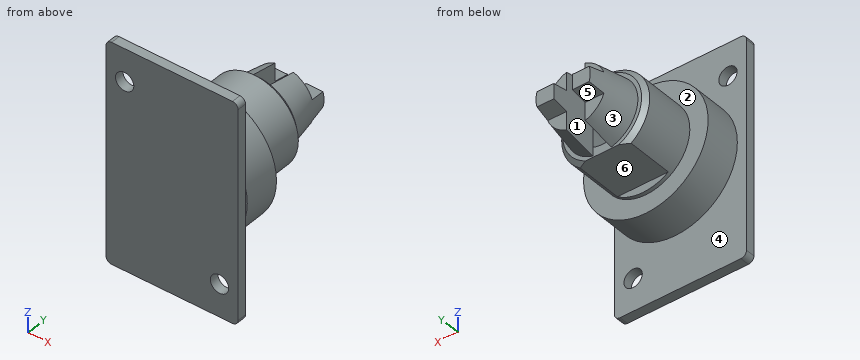
from build123d import *

# Parameters (mm, degrees)
BOSS_EXTRUDE1_DEPTH     = 1.27
SKETCH3_W               = 12
SKETCH3_H               = 12
CUT_EXTRUDE1_DEPTH      = 6.985
CUT_EXTRUDE1_DEPTH_BACK = 6.985
CUT_EXTRUDE2_DEPTH      = 12
CUT_EXTRUDE2_DEPTH_BACK = 12
SKETCH6_W               = 9.7536
SKETCH6_H               = 7.3914
CUT_EXTRUDE3_DEPTH      = 1.27
CUT_EXTRUDE3_DEPTH_BACK = 1.27
SKETCH7_R               = 1.25
CUT_EXTRUDE4_DEPTH      = 2.54
CUT_EXTRUDE4_DEPTH_BACK = 2.54
SKETCH8_R               = 1.25
CUT_EXTRUDE5_DEPTH      = 2.54
CUT_EXTRUDE5_DEPTH_BACK = 2.54


with BuildPart() as part:
    # Sketch1 → Boss-Extrude1 (new body)
    with BuildSketch(Plane(origin=(0, 0, 0), x_dir=(1, 0, 0), z_dir=(0, 1, 0))):
        with BuildLine():
            Line((-9.0043, 14.2367), (-9.0043, -14.2367))
            ThreePointArc((-9.0043, -14.2367), (-8.781115367, -14.775515367), (-8.2423, -14.9987))
            Line((-8.2423, -14.9987), (8.2423, -14.9987))
            ThreePointArc((8.2423, -14.9987), (8.781115367, -14.775515367), (9.0043, -14.2367))
            Line((9.0043, -14.2367), (9.0043, 14.2367))
            ThreePointArc((9.0043, 14.2367), (8.781115367, 14.775515367), (8.2423, 14.9987))
            Line((8.2423, 14.9987), (-8.2423, 14.9987))
            ThreePointArc((-8.2423, 14.9987), (-8.781115367, 14.775515367), (-9.0043, 14.2367))
        make_face()
    extrude(amount=BOSS_EXTRUDE1_DEPTH)

    # Sketch2 → Revolve1 (revolve)
    with BuildSketch(Plane(origin=(0, 0, 0), x_dir=(0, 0, -1), z_dir=(1, 0, 0))):
        Polygon((3.7592, 14.7066), (3.7592, 0.9398), (6.589242136, 0.9398), (6.126999938, 2.2098), (8.4963, 2.2098), (8.4963, 7.2136), (5.999999938, 7.2136), (5.999999938, 14.093100062), (5.3865, 14.7066), align=None)
    revolve(axis=Axis((0, 0.9398, 0), (0, 1, 0)))

    # Sketch3 → Cut-Extrude1 (cut, two sides)
    with BuildSketch(Plane(origin=(0, 14.7066, 0), x_dir=(1, 0, 0), z_dir=(0, 1, 0))) as cut_extrude1_sk:
        with Locations((0, 10.8966)):
            Rectangle(SKETCH3_W, SKETCH3_H)
    extrude(amount=CUT_EXTRUDE1_DEPTH, mode=Mode.SUBTRACT)
    extrude(cut_extrude1_sk.sketch, amount=-CUT_EXTRUDE1_DEPTH_BACK, mode=Mode.SUBTRACT)

    # Sketch4 → Revolve2 (revolve)
    with BuildSketch(Plane(origin=(0, 0, 0), x_dir=(0, 0, -1), z_dir=(1, 0, 0))):
        Polygon((0, 22.098), (3.573496755, 22.098), (4.8768, 14.7066), (0, 14.7066), align=None)
    revolve(axis=Axis((0, 14.7066, 0), (0, 1, 0)))

    # Sketch5 → Cut-Extrude2 (cut, two sides)
    with BuildSketch(Plane(origin=(0, 0, 0), x_dir=(0, 0, -1), z_dir=(1, 0, 0))) as cut_extrude2_sk:
        Polygon((-4.8768, 23.6982), (-4.08406916, 19.2024), (-1.418134328, 19.2024), (-1.032965672, 21.3868), (1.032965672, 21.3868), (1.418134328, 19.2024), (4.08406916, 19.2024), (4.8768, 23.6982), align=None)
    extrude(amount=CUT_EXTRUDE2_DEPTH, mode=Mode.SUBTRACT)
    extrude(cut_extrude2_sk.sketch, amount=-CUT_EXTRUDE2_DEPTH_BACK, mode=Mode.SUBTRACT)

    # Sketch6 → Cut-Extrude3 (cut, two sides)
    with BuildSketch(Plane(origin=(0, 0, 0), x_dir=(0, 0, -1), z_dir=(1, 0, 0))) as cut_extrude3_sk:
        with Locations((0, 18.4023)):
            Rectangle(SKETCH6_W, SKETCH6_H)
    extrude(amount=CUT_EXTRUDE3_DEPTH, mode=Mode.SUBTRACT)
    extrude(cut_extrude3_sk.sketch, amount=-CUT_EXTRUDE3_DEPTH_BACK, mode=Mode.SUBTRACT)

    # Sketch7 → Cut-Extrude4 (cut, two sides)
    with BuildSketch(Plane(origin=(0, 0, 0), x_dir=(1, 0, 0), z_dir=(0, 1, 0))) as cut_extrude4_sk:
        with Locations((6.4643, 10.541)):
            Circle(SKETCH7_R)
    extrude(amount=CUT_EXTRUDE4_DEPTH, mode=Mode.SUBTRACT)
    extrude(cut_extrude4_sk.sketch, amount=-CUT_EXTRUDE4_DEPTH_BACK, mode=Mode.SUBTRACT)

    # Sketch8 → Cut-Extrude5 (cut, two sides)
    with BuildSketch(Plane(origin=(0, 0, 0), x_dir=(1, 0, 0), z_dir=(0, 1, 0))) as cut_extrude5_sk:
        with Locations((-6.4643, -10.541)):
            Circle(SKETCH8_R)
    extrude(amount=CUT_EXTRUDE5_DEPTH, mode=Mode.SUBTRACT)
    extrude(cut_extrude5_sk.sketch, amount=-CUT_EXTRUDE5_DEPTH_BACK, mode=Mode.SUBTRACT)


solid = part.part
Input: part model. Units: mm. Frame: model coordinates. Face numbers are marked on the shaded views. A direction names the side the tool comes from. Coordinates: 2 decimals unless noted, no trailing zeros. Loops run counter-clockwise (first coordinate to the right, second up) from the corner with the lowest first, then second, coordinate; pieces in that order, holes last. Notation, with made-up numbers: (-23.5, 80) -> (17.5, 80) arc R19 cw to (17.5, 98) -> close; hole circle Ø11 at (27.25, -37). An arc over 180 degrees is marked (long way). One line per item, written item: value.
(1) Draft query along Y for the marked faces 4, 5 and 6. Return one class per face: pulls with the +Y half, pulls with the -Y half, needs draft (parallel to the pull), parting line crosses it, or undercut.
Answer below:
face 4: undercut
face 5: pulls with the +Y half
face 6: needs draft
(2) Ray query, line 1 along Y through (x, z) = (-4.75, -5); line 2 along Z through (x, y) = (0, 4.5); line 3 along Y through (x, z) = (2, 0). Return the intervals inside material, ascending.
Answer below:
line 1: y = 0 to 1.27, 2.21 to 7.21
line 2: z = -8.5 to -3.76, 3.76 to 8.5
line 3: y = 0 to 1.27, 14.71 to 21.39
(3) Cut plane B-B (x = 0). Output: boundary loops of the cut face in (y, z).
Answer below:
outline: (0, -15) -> (1.27, -15) -> (1.27, -6.47) -> (2.21, -6.13) -> (2.21, -8.5) -> (7.21, -8.5) -> (7.21, -6) -> (7.72, -6) -> (7.72, -4.9) -> (14.71, -4.9) -> (14.71, -3.76) -> (1.27, -3.76) -> (1.27, 3.76) -> (14.71, 3.76) -> (14.71, 5.39) -> (14.09, 6) -> (7.21, 6) -> (7.21, 8.5) -> (2.21, 8.5) -> (2.21, 6.13) -> (1.27, 6.47) -> (1.27, 15) -> (0, 15) -> close
(4) Pin query (flat end, axial travel): pin 1 Ø0.7 at (x, z) = (3, 0.5) entering from -Y; pin 2 Ø5.5 at (y, z) = (17, 1.5) entering from -X; pin 3 Ø5 at (x, y) = (3.5, 9.5) entering from -Z; pin 4 Ø1.2 at (x, z) = (2, 2.5) entering from +Y. Return the tip coordinate at first contact, or that it passes through.
Answer below:
pin 1: stops at y = 0
pin 2: stops at x = -5.71
pin 3: stops at z = -8.12
pin 4: stops at y = 19.2
(5) Cut plane D-D (y = 10.75). Output: boundary loops of the cut face in (x, z).
Answer below:
outline: (-3.47, -4.9) -> (3.47, -4.9) arc R6 ccw (long way) to start; hole circle Ø7.52 at (0, 0)
(6) Cut plane A-A (z = 11). Output: boundary loops of the cut face in (x, y), then the cut area to 3 significant figures.
Answer below:
outline: (-9, 0) -> (-7.63, 0) -> (-7.63, 1.27) -> (-9, 1.27) -> close; (-5.3, 0) -> (9, 0) -> (9, 1.27) -> (-5.3, 1.27) -> close
area: 19.9 mm2
(7) Set-up query: the marked faces 1, 2 and 3. Return all of +Z, -Z, +X, -X, +Y, -Y with unobstructed straight access to the full face (end or side cutting, diameter ignored); none if empty.
Answer below:
face 1: +Z, -Z, +Y
face 2: +Y
face 3: -X, +Y
